Verification items for the finished model (mm, model axes). Round coordinates to 2 decimals unless told otherwise and drop trailing zeros. Order: outer loops, then holes, each group sorted by start corner. A loop starts at its lowest first (then second) coordinate and runs counter-clockwise, first axis right, second up. Notation, with made-up numbers: (-29, -18.5) -> (-15, -18.5) arc R23 ccw to (-15, 9.5) -> close; hole circle Ø8 at (40.5, -1). An arc over 180 degrees is marked (long way). Put each result on its own line as item: value.
```python
from build123d import *

# Parameters (mm, degrees)
F0_R     = 5.08
F1_DEPTH = 12.7
F2_DEPTH = 25.4
F3_SIZE  = 2


with BuildPart() as f1:
    # F0 (on Front) → F1 (new body)
    with BuildSketch(Plane.XZ):
        with BuildLine():
            ThreePointArc((2.38125, -18.900586), (14.2875, -12.600391), (19.05, 0))
            ThreePointArc((19.05, 0), (14.2875, 12.600391), (2.38125, 18.900586))
            ThreePointArc((2.38125, 18.900586), (-19.05, 0), (2.38125, -18.900586))
        make_face()
        Circle(F0_R, mode=Mode.SUBTRACT)
        with BuildLine():
            ThreePointArc((2.38125, 18.900586), (14.2875, 12.600391), (19.05, 0))
            ThreePointArc((19.05, 0), (14.2875, -12.600391), (2.38125, -18.900586))
            Line((2.38125, -18.900586), (52.3875, -12.600391))
            ThreePointArc((52.3875, -12.600391), (38.1, 0), (52.3875, 12.600391))
            Line((52.3875, 12.600391), (2.38125, 18.900586))
        make_face()
        with BuildLine():
            ThreePointArc((63.5, 0), (60.325, 8.40026), (52.3875, 12.600391))
            ThreePointArc((52.3875, 12.600391), (38.1, 0), (52.3875, -12.600391))
            ThreePointArc((52.3875, -12.600391), (60.325, -8.40026), (63.5, 0))
        make_face()
        with Locations((50.8, 0)):
            Circle(F0_R, mode=Mode.SUBTRACT)
    extrude(amount=F1_DEPTH)

    # F0 (on Front) → F2 (join)
    with BuildSketch(Plane.XZ):
        with BuildLine():
            ThreePointArc((2.38125, -18.900586), (14.2875, -12.600391), (19.05, 0))
            ThreePointArc((19.05, 0), (14.2875, 12.600391), (2.38125, 18.900586))
            ThreePointArc((2.38125, 18.900586), (-19.05, 0), (2.38125, -18.900586))
        make_face()
        Circle(F0_R, mode=Mode.SUBTRACT)
    extrude(amount=F2_DEPTH)

    # F3
    f3_edges = [f1.edges().sort_by_distance(p)[0] for p in [
        (-5.08, -25.4, 0),
        (-2.38125, -25.4, 18.900586),
        (45.72, -12.7, 0),
        (-5.08, 0, 0),
        (45.72, 0, 0),
    ]]
    chamfer(f3_edges, length=F3_SIZE)


solid = f1.part
```
Item 1: Release check for a two-part mould opening along X. For faces 1 (the face through (55.49, -6.29, -1.95)), 2 (the face through (33, -12.7, 0)), 3 (the face through (27.734, -6.261, 15.706)) record: pulls with the +X half, pulls with the -X half, needs draft (parallel to the pull), parting line crosses it, or undercut.
Geometry check:
face 1: undercut
face 2: needs draft
face 3: pulls with the +X half
Item 2: Sectioned sample at A-A, the plane x = 0. Record the boundary of the cut face in (y, z).
Geometry check:
outline: (-25.4, -17.05) -> (-23.4, -19.05) -> (0, -19.05) -> (0, -7.08) -> (-2, -5.08) -> (-23.4, -5.08) -> (-25.4, -7.08) -> close; (-25.4, 7.08) -> (-23.4, 5.08) -> (-2, 5.08) -> (0, 7.08) -> (0, 19.05) -> (-23.4, 19.05) -> (-25.4, 17.05) -> close
Item 3: Material ranges on line 1 along Z through (x, y) = (0, -14.25); line 2 along X through (y, z) = (-2, 3); line 3 along Y through (x, z) = (44, -8), recorded low to high.
Geometry check:
line 1: -19.05 to -5.08, 5.08 to 19.05
line 2: -18.81 to -4.1, 4.1 to 46.7, 54.9 to 63.14
line 3: -12.7 to 0
Item 4: Sectioned sample at B-B, the plane y = -9. Record the boundary of the cut face in (x, z), then the cut area to 3 significant figures.
Geometry check:
outline: (2.38, -18.9) -> (52.39, -12.6) arc R12.7 ccw to (63.5, 0) arc R12.7 ccw to (52.39, 12.6) -> (2.38, 18.9) arc R19.05 ccw (long way) to start; hole circle Ø10.16 at (0, 0); hole circle Ø10.16 at (50.8, 0)
area: 2,290 mm2
Item 5: Depth check by flat-ended pin: pin 1 Ø1 at (x, z) = (50.5, -15) entering from -Y; pin 2 Ø12 at (x, y) = (-10, -3) entering from -Z; pin 3 Ø3 at (x, y) = (21.5, -3) entering from +Z; pin 4 Ø5 at (x, y) = (13.5, -16.5) entering from +Z. Enter the tip coordinate at first touch or a pass-through.
Geometry check:
pin 1: through
pin 2: z = -18.63
pin 3: z = 16.68
pin 4: z = 15.55
Item 6: Sectioned sample at D-D, the plane y = -20. Record the boundary of the cut face in (x, z), then the cut area to 3 significant figures.
Geometry check:
outline: (2.38, 18.9) arc R19.05 ccw (long way) to (19.05, 0) arc R19.05 ccw to start; hole circle Ø10.16 at (0, 0)
area: 1,060 mm2
Item 7: Sectioned sample at C-C, the plane x = 50.8. Record the boundary of the cut face in (y, z), then the cut area to 3 significant figures.
Geometry check:
outline: (-12.7, -12.8) -> (0, -12.8) -> (0, -7.08) -> (-2, -5.08) -> (-10.7, -5.08) -> (-12.7, -7.08) -> close; (-12.7, 7.08) -> (-10.7, 5.08) -> (-2, 5.08) -> (0, 7.08) -> (0, 12.8) -> (-12.7, 12.8) -> close
area: 188 mm2
